from build123d import *

# Parameters (mm, degrees)
BOSS_EXTRUDE1_DEPTH = 2
BOSS_EXTRUDE2_DEPTH = 54
CHAMFER1_SIZE2      = 14.230739445
CHAMFER1_SIZE       = 2


with BuildPart() as part:
    # Sketch1 → Boss-Extrude1 (new body)
    with BuildSketch(Plane(origin=(0, 0, 0), x_dir=(1, 0, 0), z_dir=(0, 1, 0))):
        with BuildLine():
            Line((-3.337814009, 14.623918683), (-10.458483896, 45.821611873))
            ThreePointArc((-10.458483896, 45.821611873), (-29.304020687, -36.746079676), (47, 0))
            Line((47, 0), (15, 0))
            ThreePointArc((15, 0), (9.352347028, 11.727472237), (-3.337814009, 14.623918683))
        make_face()
    extrude(amount=BOSS_EXTRUDE1_DEPTH)

    # Sketch2 → Boss-Extrude2 (add)
    with BuildSketch(Plane(origin=(0, 2, 0), x_dir=(1, 0, 0), z_dir=(0, 1, 0))):
        with BuildLine():
            Line((28.057041084, 35.182416711), (29.304020687, 36.746079676))
            ThreePointArc((29.304020687, 36.746079676), (-42.345536791, -20.392535739), (47, 0))
            Line((47, 0), (45, 0))
            ThreePointArc((45, 0), (-40.543599056, -19.52476826), (28.057041084, 35.182416711))
        make_face()
    extrude(amount=BOSS_EXTRUDE2_DEPTH)

    # Chamfer1
    chamfer1_edges = [part.edges().sort_by_distance(p)[0] for p in [
        (30, 2, 0),
    ]]
    chamfer1_side = [part.faces().sort_by_distance(p)[0] for p in [
        (30, 1.96, 0),
    ]]
    chamfer(chamfer1_edges, length=CHAMFER1_SIZE - 0.0001, length2=CHAMFER1_SIZE2 - 0.0001, reference=chamfer1_side[0])  # a hair under: the kernel refuses the full size


solid = part.part
The model under review builds one solid part; all positions refer to its coordinate system, in mm. A direction names the side the tool comes from. Coordinates: 2 decimals unless noted, no trailing zeros. Write each loop counter-clockwise with the first axis right and the second up, starting at its lowest first coordinate (ties: lowest second). Pieces come first, ordered by that corner, then holes. Notation, with made-up numbers: (-28.5, 33) - (28.5, 33) arc R8 ccw to (28.5, 48) - close; hole circle Ø6 at (76.25, 50.25). An arc over 180 degrees is marked (long way). Answer as a JSON object with one key per item and string values. Group by question number.
1. Add section A-A (x = 0). Give the boundary of the cut face in (y, z).
2. Add section C-C (z = -23.5). Give the boundary of the cut face in (x, y).
3. Clearance check with flat-ended pins moving along their axes: pin 1 Ø1 at (x, z) = (1.5, 18) entering from +Y; pin 2 Ø12 at (x, y) = (-5.5, 8) entering from -Z; pin 3 Ø6 at (x, y) = (21, 45) entering from -Z. State where each tip first meets the part, or that it passes through.
4. To check wall thickness, follow probe 1 along Z at (x, y) = (0, 22); probe 2 along Y at (x, z) = (-32.5, -23.5); probe 3 along Z at (x, y) = (-30, 10). State the ranges of each line that lie inside material, in increasing order.
5. Add section D-D (y = 39). Give the boundary of the cut face in (x, z), plus the area to 3 significant figures.
6. Machinability: for faces 1 (the face through (11, 2, -44)), 2 (the face through (45.3, 27.9, 0)), 3 (the face through (-12, 2, 10)), which of the approach directions +Z, -Z, +X, -X, +Y, -Y give a long, thin tool a straight path to every point of the face, cutting with its end or side? Answer none if there is none.
Findings:
{
 "1": {"outline": "(0, -15) - (2, -15) - (2, 45) - (56, 45) - (56, 47) - (0, 47) - close; (2, -47) - (56, -47) - (56, -45) - (2, -45) - close"},
 "2": {"outline": "(-40.7, 0) - (-5.36, 0) - (-5.36, 2) - (-38.38, 2) - (-38.38, 56) - (-40.7, 56) - close"},
 "3": {"pin 1": "y = 2", "pin 2": "z = -47", "pin 3": "z = -43.42"},
 "4": {"probe 1": "-47 to -45, 45 to 47", "probe 2": "0 to 2", "probe 3": "-36.18 to -33.54, 33.54 to 36.18"},
 "5": {"outline": "(28.06, -35.18) arc R45 cw (long way) to (45, 0) - (47, 0) arc R47 ccw (long way) to (29.3, -36.75) - close", "area": "495 mm²"},
 "6": {"face 1": "-Z, +X, -Y", "face 2": "-Z, +X, +Y, -Y", "face 3": "+Y"}
}
